Verification items for the finished model (mm, model axes). Face numbers are marked on the shaded views. A direction names the side the tool comes from. Coordinates: 2 decimals unless noted, no trailing zeros. Order: outer loops, then holes, each group sorted by start corner. A loop starts at its lowest first (then second) coordinate and runs counter-clockwise, first axis right, second up.
Q1. Cross-section at B-B, the plane z = 20. Record the boundary of the cut face in (x, y), and give its area (3 significant figures).
Q2. Cross-section at A-A, the plane x = -19.5. Record the boundary of the cut face in (y, z).
Q3. Thickness scan on line 1 (X direction, y = 3, z = 18); line 2 (Y direction, x = 9, z = 31.5); line 3 (X direction, y = 44.1, z = 20). Record the ranges inside material, lowest first.
Q4. Depth check by flat-ended pin: P1, Ø9.5, axis at y = 32.5, z = 24, coming from the +X side; P2, Ø4, axis at x = 16, z = 18, coming from the +Y side; P3, Ø4, axis at y = 32, z = 9.5, coming from the -X side; P4, Ø6, axis at x = 15.5, z = 21, coming from the +Y side. Enter the tip coordinate at first touch or a pass-through.
Q5. Draft check along Z on the marked faces 6, 7 and 8. Enter one of: pulls with the +Z half, pulls with the -Z half, needs draft (parallel to the pull), parting line crosses it, or undercut.
Q6. Set-up check for the marked faces 1, 2, 3, 4 and 5: record each of +Z, -Z, +X, -X, +Y, -Y from which the full face is reachable in a straight line by a thin tool's end or side.
Q7. Cross-section at C-C, the plane z = 6. Record the boundary of the cut face in (x, y).
from build123d import *

# Parameters (mm, degrees)
BOSS_EXTRUDE1_DEPTH = 36
SKETCH3_R           = 3.5
CUT_EXTRUDE1_DEPTH  = 32
SKETCH2_R           = 8.2
CUT_EXTRUDE2_DEPTH  = 32
CUT_EXTRUDE3_DEPTH  = 6
BOSS_EXTRUDE3_DEPTH = 4
CUT_EXTRUDE4_DEPTH  = 3.3
FILLET1_R           = 4
FILLET4_R           = 2


with BuildPart() as part:
    # Sketch1 → Boss-Extrude1 (new body)
    with BuildSketch(Plane.XY):
        Polygon((0, 0), (0, 40), (-30, 40), (-30, 47), (6, 47), (6, 12), (26, 12), (26, 0), align=None)
    extrude(amount=BOSS_EXTRUDE1_DEPTH)

    # Sketch3 → Cut-Extrude1 (cut)
    with BuildSketch(Plane(origin=(0, 12, 0), x_dir=(1, 0, 0), z_dir=(0, 1, 0))):
        with Locations(Location((16, -18, 0), (0, 0, 270))):
            Circle(SKETCH3_R)
    extrude(amount=-CUT_EXTRUDE1_DEPTH, mode=Mode.SUBTRACT)

    # Sketch2 → Cut-Extrude2 (cut)
    with BuildSketch(Plane(origin=(0, 47, 0), x_dir=(1, 0, 0), z_dir=(0, 1, 0))):
        with Locations(Location((-14, -20, 0), (0, 0, 270))):
            Circle(SKETCH2_R)
    extrude(amount=-CUT_EXTRUDE2_DEPTH, mode=Mode.SUBTRACT)

    # Sketch4 → Cut-Extrude3 (cut)
    with BuildSketch(Plane(origin=(0, 12, 0), x_dir=(1, 0, 0), z_dir=(0, 1, 0))):
        Polygon((16, -24.639528096), (21.75, -21.319764048), (21.75, -14.680235952), (16, -11.360471904), (10.25, -14.680235952), (10.25, -21.319764048), align=None)
    extrude(amount=-CUT_EXTRUDE3_DEPTH, mode=Mode.SUBTRACT)

    # Sketch5 → Boss-Extrude3 (add)
    with BuildSketch(Plane(origin=(0, 0, 0), x_dir=(-1, 0, 0), z_dir=(0, 0, -1))):
        Polygon((-26, 12), (-6, 32), (-6, 12), align=None)
        Polygon((0, 10), (0, 40), (30, 40), align=None)
    extrude(amount=-BOSS_EXTRUDE3_DEPTH)

    # Sketch6 → Cut-Extrude4 (cut)
    with BuildSketch(Plane.XZ.offset(-40)):
        Polygon((-14, 4.988893001), (-1, 12.494446501), (-1, 27.505553499), (-14, 35.011106999), (-27, 27.505553499), (-27, 12.494446501), align=None)
    extrude(amount=-CUT_EXTRUDE4_DEPTH, mode=Mode.SUBTRACT)

    # Fillet1
    fillet1_edges = [part.edges().sort_by_distance(p)[0] for p in [
        (26, 6, 0),
        (-30, 43.5, 36),
        (26, 6, 36),
        (-30, 43.5, 0),
    ]]
    fillet(fillet1_edges, radius=FILLET1_R)

    # Fillet4
    fillet4_edges = [part.edges().sort_by_distance(p)[0] for p in [
        (26, 0, 18),
        (24.828427125, 0, 1.171572875),
        (24.828427125, 0, 34.828427125),
        (-30, 47, 18),
        (11, 0, 0),
        (-28.828427125, 47, 1.171572875),
        (-28.828427125, 47, 34.828427125),
        (0, 0, 18),
        (6, 47, 18),
        (6, 29.5, 36),
        (-10, 47, 36),
        (0, 20, 36),
        (11, 0, 36),
        (6, 39.5, 0),
        (-10, 47, 0),
    ]]
    fillet(fillet4_edges, radius=FILLET4_R)


solid = part.part
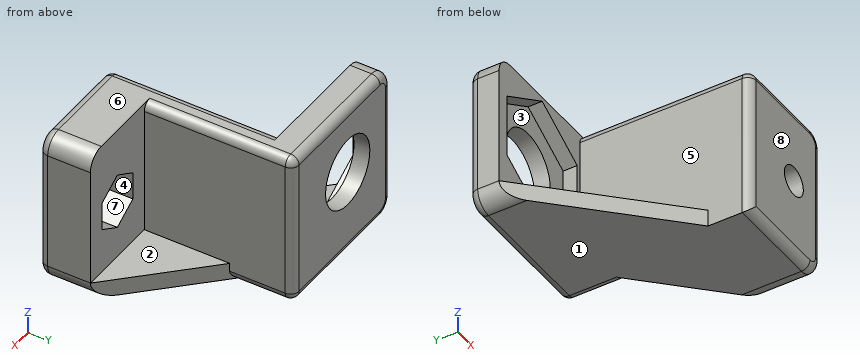
Check values:
1. outline: (-30, 40) - (-27, 40) - (-27, 43.3) - (-22.2, 43.3) - (-22.2, 47) - (-28, 47) arc R2 ccw to (-30, 45) - close; (-5.8, 43.3) - (-1, 43.3) - (-1, 40) - (0, 40) - (0, 2) arc R2 ccw to (2, 0) - (13.13, 0) - (13.13, 6) - (10.25, 6) - (10.25, 12) - (6, 12) - (6, 45) arc R2 ccw to (4, 47) - (-5.8, 47) - close; (18.87, 0) - (24, 0) arc R2 ccw to (26, 2) - (26, 12) - (21.75, 12) - (21.75, 6) - (18.87, 6) - close
1. area: 479 mm2
2. outline: (29.5, 0) - (45, 0) arc R2 ccw to (47, 2) - (47, 13.92) - (43.3, 13.92) - (43.3, 8.16) - (40, 8.16) - (40, 4) - (29.5, 4) - close; (40, 31.84) - (43.3, 31.84) - (43.3, 26.08) - (47, 26.08) - (47, 34) arc R2 ccw to (45, 36) - (40, 36) - close
3. line 1: x = 0 to 12.5, 19.5 to 26
3. line 2: y = 0 to 12
3. line 3: x = -30 to -22.2, -5.8 to 6
4. P1: stops at x = 6
4. P2: passes through
4. P3: stops at x = 0
4. P4: stops at y = 12
5. face 6: pulls with the +Z half
5. face 7: undercut
5. face 8: needs draft
6. face 1: -Z, +X, -X, +Y, -Y
6. face 2: +Z, +X, +Y
6. face 3: -Y
6. face 4: +Y
6. face 5: +Z, -X, -Y
7. outline: (-30, 40) - (-15.75, 40) - (-15.75, 43.3) - (-12.25, 43.3) - (-12.25, 40) - (0, 40) - (0, 2) arc R2 ccw to (2, 0) - (24, 0) arc R2 ccw to (26, 2) - (26, 12) - (6, 12) - (6, 45) arc R2 ccw to (4, 47) - (-28, 47) arc R2 ccw to (-30, 45) - close
